from build123d import *

# Parameters (mm, degrees)
F0_W     = 155
F0_H     = 15
F1_DEPTH = 4
F2_W     = 8
F2_H     = 15
F3_DEPTH = 8
F4_W     = 8
F4_H     = 6
F4_H_2   = 5.5
F5_DEPTH = 3
F6_R     = 1


# Not quite as in the source:
# - a feature names something its author has since deleted; it is built from what else it names


with BuildPart() as f1:
    # F0 (on Front) → F1 (new body)
    with BuildSketch(Plane.XZ):
        Rectangle(F0_W, F0_H)
        with BuildLine():
            Line((-72.25, -2.5), (-72.25, 2.5))
            ThreePointArc((-72.25, 2.5), (-70, 4.75), (-67.75, 2.5))
            Line((-67.75, 2.5), (-67.75, -2.5))
            ThreePointArc((-67.75, -2.5), (-70, -4.75), (-72.25, -2.5))
        make_face(mode=Mode.SUBTRACT)
        with BuildLine():
            ThreePointArc((67.75, 2.5), (70, 4.75), (72.25, 2.5))
            Line((72.25, 2.5), (72.25, -2.5))
            ThreePointArc((72.25, -2.5), (70, -4.75), (67.75, -2.5))
            Line((67.75, -2.5), (67.75, 2.5))
        make_face(mode=Mode.SUBTRACT)
    extrude(amount=F1_DEPTH)

    # F2 (on face) → F3 (join)
    with BuildSketch(Plane.XZ.offset(4)):
        with Locations((-59, 0)):
            Rectangle(F2_W, F2_H)
        with Locations((59, 0)):
            Rectangle(F2_W, F2_H)
    extrude(amount=F3_DEPTH)

    # F4 (on face) → F5 (join)
    with BuildSketch(Plane(origin=(0, 0, -7.5), x_dir=(1, 0, 0), z_dir=(0, 0, -1))):
        with Locations((-59, 9)):
            Rectangle(F4_W, F4_H)
        with Locations((59, 9.25)):
            Rectangle(F4_W, F4_H_2)
    extrude(amount=F5_DEPTH)

    # F6
    f6_edges = [f1.edges().sort_by_distance(p)[0] for p in [
        (55, -4, 0),
        (-55, -4, 0),
        (63, -4, 0),
        (-63, -4, 0),
    ]]
    fillet(f6_edges, radius=F6_R)


solid = f1.part
Input: part model. Units: mm. Frame: model coordinates. A direction names the side the tool comes from. Give positions to 0.01 mm unless a question says otherwise; leave off trailing zeros. Write each loop counter-clockwise with the first axis right and the second up, starting at its lowest first coordinate (ties: lowest second). Pieces come first, ordered by that corner, then holes.
Q1. Set-up query: faces 1 (the face through (-63, -8, -1)), 2 (the face through (-69.95, -1.97, -4.75)), 3 (the face through (55, -8, -2)), 4 (the face through (5, -3, 7.5)), 5 (the face through (59, -6.5, -9)). Return all of +Z, -Z, +X, -X, +Y, -Y with unobstructed straight access to the full face (end or side cutting, diameter ignored); none if empty.
Q2. Material intervals for probe 1 along X at (y, z) = (-2.5, -0.75); probe 2 along X at (y, z) = (-8.25, 1); probe 3 along X at (y, z) = (-0.5, 3.5), sorted ascending.
Q3. First-contact query: P1, Ø2, axis at y = -7.5, z = -1, coming from the -X side; P2, Ø7, axis at x = -9.5, y = -3, coming from the -Z side; P3, Ø2, axis at y = -7, z = -1.5, coming from the +X side. Flat tips, straight axial feed; report the tip coordinate or a pass-through.
Q4. Section D-D, the plane x = 47. Output: boundary loops of the cut face in (y, z), plus the area to 3 significant figures.
Q5. Section C-C, the plane z = 0.25. Output: boundary loops of the cut face in (x, y).
Q6. Section A-A, the plane x = -70. Output: boundary loops of the cut face in (y, z), plus the area to 3 significant figures.
Q7. Section B-B, the plane y = -8. Output: boundary loops of the cut face in (x, z), plus the area to 3 significant figures.
Q8. Pull-direction query (Z, two-part tool) for faces 6 (the face through (59, -9, -10.5)), 7 (the face through (69.95, -1.97, 4.75)), 8 (the face through (-59, -6, -9)); classes: pulls with the +Z half, pulls with the -Z half, needs draft (parallel to the pull), parting line crosses it, or undercut.
Filled in:
1. face 1: +Z, -Z, -X, -Y
1. face 2: +Y, -Y
1. face 3: +Z, -Z, -Y
1. face 4: +Z, +X, -X, +Y, -Y
1. face 5: -Z, +X, +Y
2. probe 1: x = -77.5 to -72.25, -67.75 to 67.75, 72.25 to 77.5
2. probe 2: x = -63 to -55, 55 to 63
2. probe 3: x = -77.5 to -72.02, -67.98 to 67.98, 72.02 to 77.5
3. P1: stops at x = -63
3. P2: stops at z = -7.5
3. P3: stops at x = 63
4. outline: (-4, -7.5) - (0, -7.5) - (0, 7.5) - (-4, 7.5) - close
4. area: 60.0 mm2
5. outline: (-77.5, -4) - (-72.25, -4) - (-72.25, 0) - (-77.5, 0) - close; (-67.75, -4) - (-64, -4) arc R1 cw to (-63, -5) - (-63, -12) - (-55, -12) - (-55, -5) arc R1 cw to (-54, -4) - (54, -4) arc R1 cw to (55, -5) - (55, -12) - (63, -12) - (63, -5) arc R1 cw to (64, -4) - (67.75, -4) - (67.75, 0) - (-67.75, 0) - close; (72.25, -4) - (77.5, -4) - (77.5, 0) - (72.25, 0) - close
6. outline: (-4, -7.5) - (0, -7.5) - (0, -4.75) - (-4, -4.75) - close; (-4, 4.75) - (0, 4.75) - (0, 7.5) - (-4, 7.5) - close
6. area: 22.0 mm2
7. outline: (-63, -10.5) - (-55, -10.5) - (-55, 7.5) - (-63, 7.5) - close; (55, -10.5) - (63, -10.5) - (63, 7.5) - (55, 7.5) - close
7. area: 288 mm2
8. face 6: pulls with the -Z half
8. face 7: undercut
8. face 8: needs draft
